Part model, mm, in its own coordinate system. A direction names the side the tool comes from. Coordinates: 2 decimals unless noted, no trailing zeros. Write each loop counter-clockwise with the first axis right and the second up, starting at its lowest first coordinate (ties: lowest second). Pieces come first, ordered by that corner, then holes. Notation, with made-up numbers: (9.5, 44) -> (32.5, 44) arc R16 ccw to (32.5, 71) -> close; hole circle Ø1 at (70.25, -20). An arc over 180 degrees is marked (long way). One line per question, with ' | ' between items. Start each with the question number.
Item 1: Saw through at C-C (y = 31). List the corners of the cut face in (x, z), and give its area (3 significant figures).
Item 2: Saw through at D-D (x = -6). List the corners of the cut face in (y, z).
Item 3: Saw through at B-B (x = 0). List the corners of the cut face in (y, z).
Item 4: 3-axis set-ups, long thin cutter, end or side, ignore diameter. For faces 1 (the flat face through (0, -30, -50)), 2 (the flat face through (0, 20, -2)): which of +Z, -Z, +X, -X, +Y, -Y reach the whole face in a straight line?
Item 5: Two-plate mould, pull along Y, no slides. Class faces 3 (the flat face through (0, 0, 30)), 4 (the cylindrical face through (-1.953, 30.14, -11.217)), 5 (the flat face through (0, 40, 1)), 6 (the flat face through (0, -40, 1)): pulls with the +Y half, pulls with the -Y half, needs draft (parallel to the pull), parting line crosses it, or undercut.
Item 6: Probe probe 1 along Y at (x, z) = (-16, 14); probe 2 along Z at (x, y) = (0, -29.75); probe 3 along Z at (x, y) = (18, 17). List the from-to ranges inside material, lowest first. Write a range as [from, to].
Item 7: Pin check, flat tip, straight feed: pin 1 (3 mm diameter, centred on x = 7, y = -11.5, fed in from -Z). Stop position of the tip, or through.
Item 8: Saw through at A-A (z = -3.5). List the corners of the cut face in (x, y).
from build123d import *

# Parameters (mm, degrees)
F0_W     = 40
F0_H     = 100
F0_R     = 15
F1_DEPTH = 40
F2_W     = 40
F2_H     = 80
F3_DEPTH = 60


with BuildPart() as f1:
    # F0 (on Front) → F1 (new body, symmetric)
    with BuildSketch(Plane.XZ):
        Rectangle(F0_W, F0_H)
        with Locations((0, -26.0889567435)):
            Circle(F0_R, mode=Mode.SUBTRACT)
    extrude(amount=F1_DEPTH, both=True)

    # F2 (on face) → F3 (cut, symmetric)
    with BuildSketch(Plane(origin=(-20, 0, 0), x_dir=(0, -1, 0), z_dir=(-1, 0, 0))):
        with Locations((0, -10)):
            Rectangle(F2_W, F2_H)
    extrude(amount=F3_DEPTH, both=True, mode=Mode.SUBTRACT)


solid = f1.part
From the geometry:
1) outline: (-20, -50) -> (20, -50) -> (20, 50) -> (-20, 50) -> close; hole circle Ø30 at (0, -26.09) | area: 3,290 mm2
2) outline: (-40, -50) -> (-20, -50) -> (-20, -39.84) -> (-40, -39.84) -> close; (-40, -12.34) -> (-20, -12.34) -> (-20, 30) -> (20, 30) -> (20, -12.34) -> (40, -12.34) -> (40, 50) -> (-40, 50) -> close; (20, -50) -> (40, -50) -> (40, -39.84) -> (20, -39.84) -> close
3) outline: (-40, -50) -> (-20, -50) -> (-20, -41.09) -> (-40, -41.09) -> close; (-40, -11.09) -> (-20, -11.09) -> (-20, 30) -> (20, 30) -> (20, -11.09) -> (40, -11.09) -> (40, 50) -> (-40, 50) -> close; (20, -50) -> (40, -50) -> (40, -41.09) -> (20, -41.09) -> close
4) face 1: -Z, +X, -X, +Y, -Y | face 2: -Z, +X, -X
5) face 3: undercut | face 4: needs draft | face 5: pulls with the +Y half | face 6: pulls with the -Y half
6) probe 1: [-40, -20], [20, 40] | probe 2: [-50, -41.09], [-11.09, 50] | probe 3: [30, 50]
7) pin 1: z = 30
8) outline: (-20, -40) -> (20, -40) -> (20, -20) -> (-20, -20) -> close; (-20, 20) -> (20, 20) -> (20, 40) -> (-20, 40) -> close
